```python
from build123d import *

# Parameters (mm, degrees)
SKETCH1_R           = 124
BOSS_EXTRUDE1_DEPTH = 6.35
SKETCH6_R           = 2.5527
CUT_EXTRUDE1_DEPTH  = 176.477413076
SKETCH8_R           = 11
CUT_EXTRUDE3_DEPTH  = 176.477413076
SKETCH9_R           = 2.45
CUT_EXTRUDE4_DEPTH  = 176.477413076
SKETCH12_R          = 1.45
CUT_EXTRUDE5_DEPTH  = 176.477413076
SKETCH13_R          = 54
CUT_EXTRUDE6_DEPTH  = 176.477413076


with BuildPart() as part:
    # Sketch1 → Boss-Extrude1 (new body)
    with BuildSketch(Plane(origin=(0, 0, 0), x_dir=(1, 0, 0), z_dir=(0, 1, 0))):
        with Locations(Location((0, 0, 0), (0, 0, 270))):
            Circle(SKETCH1_R)
    extrude(amount=BOSS_EXTRUDE1_DEPTH)

    # Sketch6 → Cut-Extrude1 (cut, through all)
    with BuildSketch(Plane.XZ):
        with Locations(Location((-109.204648421, 41.27165811, 0), (0, 0, 270))):
            Circle(SKETCH6_R)
        with Locations(Location((-106.602870566, -47.590261473, 0), (0, 0, 270))):
            Circle(SKETCH6_R)
        with Locations(Location((109.204648421, -41.27165811, 0), (0, 0, 270))):
            Circle(SKETCH6_R)
        with Locations(Location((106.602870566, 47.590261473, 0), (0, 0, 270))):
            Circle(SKETCH6_R)
        with Locations(Location((41.27165811, 109.204648421, 0), (0, 0, 270))):
            Circle(SKETCH6_R)
        with Locations(Location((-47.590261473, 106.602870566, 0), (0, 0, 270))):
            Circle(SKETCH6_R)
        with Locations(Location((-41.27165811, -109.204648421, 0), (0, 0, 270))):
            Circle(SKETCH6_R)
        with Locations(Location((47.590261473, -106.602870566, 0), (0, 0, 270))):
            Circle(SKETCH6_R)
    extrude(amount=-CUT_EXTRUDE1_DEPTH, mode=Mode.SUBTRACT)

    # Sketch8 → Cut-Extrude3 (cut, through all)
    with BuildSketch(Plane(origin=(0, 6.35, 0), x_dir=(1, 0, 0), z_dir=(0, 1, 0))):
        with Locations(Location((0, 0, 0), (0, 0, 270))):
            Circle(SKETCH8_R)
    extrude(amount=-CUT_EXTRUDE3_DEPTH, mode=Mode.SUBTRACT)

    # Sketch9 → Cut-Extrude4 (cut, through all)
    with BuildSketch(Plane(origin=(0, 6.35, 0), x_dir=(1, 0, 0), z_dir=(0, 1, 0))):
        with Locations(Location((-15.112143296, -8.725, 0), (0, 0, 270))):
            Circle(SKETCH9_R)
        with Locations(Location((0, 17.45, 0), (0, 0, 270))):
            Circle(SKETCH9_R)
        with Locations(Location((15.112143296, -8.725, 0), (0, 0, 270))):
            Circle(SKETCH9_R)
    extrude(amount=-CUT_EXTRUDE4_DEPTH, mode=Mode.SUBTRACT)

    # Sketch12 → Cut-Extrude5 (cut, through all)
    with BuildSketch(Plane(origin=(0, 6.35, 0), x_dir=(1, 0, 0), z_dir=(0, 1, 0))):
        with Locations(Location((0, 30, 0), (0, 0, 270))):
            Circle(SKETCH12_R)
        with Locations(Location((0, 60, 0), (0, 0, 270))):
            Circle(SKETCH12_R)
        with Locations(Location((0, 90, 0), (0, 0, 270))):
            Circle(SKETCH12_R)
        with Locations(Location((11.480502971, 27.716385975, 0), (0, 0, 270))):
            Circle(SKETCH12_R)
        with Locations(Location((21.213203436, 21.213203436, 0), (0, 0, 270))):
            Circle(SKETCH12_R)
        with Locations(Location((27.716385975, 11.480502971, 0), (0, 0, 270))):
            Circle(SKETCH12_R)
        with Locations(Location((30, 0, 0), (0, 0, 270))):
            Circle(SKETCH12_R)
        with Locations(Location((27.716385975, -11.480502971, 0), (0, 0, 270))):
            Circle(SKETCH12_R)
        with Locations(Location((21.213203436, -21.213203436, 0), (0, 0, 270))):
            Circle(SKETCH12_R)
        with Locations(Location((11.480502971, -27.716385975, 0), (0, 0, 270))):
            Circle(SKETCH12_R)
        with Locations(Location((0, -30, 0), (0, 0, 270))):
            Circle(SKETCH12_R)
        with Locations(Location((-11.480502971, -27.716385975, 0), (0, 0, 270))):
            Circle(SKETCH12_R)
        with Locations(Location((-21.213203436, -21.213203436, 0), (0, 0, 270))):
            Circle(SKETCH12_R)
        with Locations(Location((-27.716385975, -11.480502971, 0), (0, 0, 270))):
            Circle(SKETCH12_R)
        with Locations(Location((-30, 0, 0), (0, 0, 270))):
            Circle(SKETCH12_R)
        with Locations(Location((-27.716385975, 11.480502971, 0), (0, 0, 270))):
            Circle(SKETCH12_R)
        with Locations(Location((-21.213203436, 21.213203436, 0), (0, 0, 270))):
            Circle(SKETCH12_R)
        with Locations(Location((-11.480502971, 27.716385975, 0), (0, 0, 270))):
            Circle(SKETCH12_R)
        with Locations(Location((11.705419321, 58.847116824, 0), (0, 0, 270))):
            Circle(SKETCH12_R)
        with Locations(Location((22.961005942, 55.432771951, 0), (0, 0, 270))):
            Circle(SKETCH12_R)
        with Locations(Location((33.334213981, 49.888176738, 0), (0, 0, 270))):
            Circle(SKETCH12_R)
        with Locations(Location((42.426406871, 42.426406871, 0), (0, 0, 270))):
            Circle(SKETCH12_R)
        with Locations(Location((49.888176738, 33.334213981, 0), (0, 0, 270))):
            Circle(SKETCH12_R)
        with Locations(Location((55.432771951, 22.961005942, 0), (0, 0, 270))):
            Circle(SKETCH12_R)
        with Locations(Location((58.847116824, 11.705419321, 0), (0, 0, 270))):
            Circle(SKETCH12_R)
        with Locations(Location((60, 0, 0), (0, 0, 270))):
            Circle(SKETCH12_R)
        with Locations(Location((58.847116824, -11.705419321, 0), (0, 0, 270))):
            Circle(SKETCH12_R)
        with Locations(Location((55.432771951, -22.961005942, 0), (0, 0, 270))):
            Circle(SKETCH12_R)
        with Locations(Location((49.888176738, -33.334213981, 0), (0, 0, 270))):
            Circle(SKETCH12_R)
        with Locations(Location((42.426406871, -42.426406871, 0), (0, 0, 270))):
            Circle(SKETCH12_R)
        with Locations(Location((33.334213981, -49.888176738, 0), (0, 0, 270))):
            Circle(SKETCH12_R)
        with Locations(Location((22.961005942, -55.432771951, 0), (0, 0, 270))):
            Circle(SKETCH12_R)
        with Locations(Location((11.705419321, -58.847116824, 0), (0, 0, 270))):
            Circle(SKETCH12_R)
        with Locations(Location((0, -60, 0), (0, 0, 270))):
            Circle(SKETCH12_R)
        with Locations(Location((-11.705419321, -58.847116824, 0), (0, 0, 270))):
            Circle(SKETCH12_R)
        with Locations(Location((-22.961005942, -55.432771951, 0), (0, 0, 270))):
            Circle(SKETCH12_R)
        with Locations(Location((-33.334213981, -49.888176738, 0), (0, 0, 270))):
            Circle(SKETCH12_R)
        with Locations(Location((-42.426406871, -42.426406871, 0), (0, 0, 270))):
            Circle(SKETCH12_R)
        with Locations(Location((-49.888176738, -33.334213981, 0), (0, 0, 270))):
            Circle(SKETCH12_R)
        with Locations(Location((-55.432771951, -22.961005942, 0), (0, 0, 270))):
            Circle(SKETCH12_R)
        with Locations(Location((-58.847116824, -11.705419321, 0), (0, 0, 270))):
            Circle(SKETCH12_R)
        with Locations(Location((-60, 0, 0), (0, 0, 270))):
            Circle(SKETCH12_R)
        with Locations(Location((-58.847116824, 11.705419321, 0), (0, 0, 270))):
            Circle(SKETCH12_R)
        with Locations(Location((-55.432771951, 22.961005942, 0), (0, 0, 270))):
            Circle(SKETCH12_R)
        with Locations(Location((-49.888176738, 33.334213981, 0), (0, 0, 270))):
            Circle(SKETCH12_R)
        with Locations(Location((-42.426406871, 42.426406871, 0), (0, 0, 270))):
            Circle(SKETCH12_R)
        with Locations(Location((-33.334213981, 49.888176738, 0), (0, 0, 270))):
            Circle(SKETCH12_R)
        with Locations(Location((-22.961005942, 55.432771951, 0), (0, 0, 270))):
            Circle(SKETCH12_R)
        with Locations(Location((-11.705419321, 58.847116824, 0), (0, 0, 270))):
            Circle(SKETCH12_R)
        with Locations(Location((14.079101854, 88.891950654, 0), (0, 0, 270))):
            Circle(SKETCH12_R)
        with Locations(Location((27.811529494, 85.595086467, 0), (0, 0, 270))):
            Circle(SKETCH12_R)
        with Locations(Location((40.859144977, 80.190587177, 0), (0, 0, 270))):
            Circle(SKETCH12_R)
        with Locations(Location((52.900672706, 72.811529494, 0), (0, 0, 270))):
            Circle(SKETCH12_R)
        with Locations(Location((63.639610307, 63.639610307, 0), (0, 0, 270))):
            Circle(SKETCH12_R)
        with Locations(Location((72.811529494, 52.900672706, 0), (0, 0, 270))):
            Circle(SKETCH12_R)
        with Locations(Location((80.190587177, 40.859144977, 0), (0, 0, 270))):
            Circle(SKETCH12_R)
        with Locations(Location((85.595086467, 27.811529494, 0), (0, 0, 270))):
            Circle(SKETCH12_R)
        with Locations(Location((88.891950654, 14.079101854, 0), (0, 0, 270))):
            Circle(SKETCH12_R)
        with Locations(Location((90, 0, 0), (0, 0, 270))):
            Circle(SKETCH12_R)
        with Locations(Location((88.891950654, -14.079101854, 0), (0, 0, 270))):
            Circle(SKETCH12_R)
        with Locations(Location((85.595086467, -27.811529494, 0), (0, 0, 270))):
            Circle(SKETCH12_R)
        with Locations(Location((80.190587177, -40.859144977, 0), (0, 0, 270))):
            Circle(SKETCH12_R)
        with Locations(Location((72.811529494, -52.900672706, 0), (0, 0, 270))):
            Circle(SKETCH12_R)
        with Locations(Location((63.639610307, -63.639610307, 0), (0, 0, 270))):
            Circle(SKETCH12_R)
        with Locations(Location((52.900672706, -72.811529494, 0), (0, 0, 270))):
            Circle(SKETCH12_R)
        with Locations(Location((40.859144977, -80.190587177, 0), (0, 0, 270))):
            Circle(SKETCH12_R)
        with Locations(Location((27.811529494, -85.595086467, 0), (0, 0, 270))):
            Circle(SKETCH12_R)
        with Locations(Location((14.079101854, -88.891950654, 0), (0, 0, 270))):
            Circle(SKETCH12_R)
        with Locations(Location((0, -90, 0), (0, 0, 270))):
            Circle(SKETCH12_R)
        with Locations(Location((-14.079101854, -88.891950654, 0), (0, 0, 270))):
            Circle(SKETCH12_R)
        with Locations(Location((-27.811529494, -85.595086467, 0), (0, 0, 270))):
            Circle(SKETCH12_R)
        with Locations(Location((-40.859144977, -80.190587177, 0), (0, 0, 270))):
            Circle(SKETCH12_R)
        with Locations(Location((-52.900672706, -72.811529494, 0), (0, 0, 270))):
            Circle(SKETCH12_R)
        with Locations(Location((-63.639610307, -63.639610307, 0), (0, 0, 270))):
            Circle(SKETCH12_R)
        with Locations(Location((-72.811529494, -52.900672706, 0), (0, 0, 270))):
            Circle(SKETCH12_R)
        with Locations(Location((-80.190587177, -40.859144977, 0), (0, 0, 270))):
            Circle(SKETCH12_R)
        with Locations(Location((-85.595086467, -27.811529494, 0), (0, 0, 270))):
            Circle(SKETCH12_R)
        with Locations(Location((-88.891950654, -14.079101854, 0), (0, 0, 270))):
            Circle(SKETCH12_R)
        with Locations(Location((-90, 0, 0), (0, 0, 270))):
            Circle(SKETCH12_R)
        with Locations(Location((-88.891950654, 14.079101854, 0), (0, 0, 270))):
            Circle(SKETCH12_R)
        with Locations(Location((-85.595086467, 27.811529494, 0), (0, 0, 270))):
            Circle(SKETCH12_R)
        with Locations(Location((-80.190587177, 40.859144977, 0), (0, 0, 270))):
            Circle(SKETCH12_R)
        with Locations(Location((-72.811529494, 52.900672706, 0), (0, 0, 270))):
            Circle(SKETCH12_R)
        with Locations(Location((-63.639610307, 63.639610307, 0), (0, 0, 270))):
            Circle(SKETCH12_R)
        with Locations(Location((-52.900672706, 72.811529494, 0), (0, 0, 270))):
            Circle(SKETCH12_R)
        with Locations(Location((-40.859144977, 80.190587177, 0), (0, 0, 270))):
            Circle(SKETCH12_R)
        with Locations(Location((-27.811529494, 85.595086467, 0), (0, 0, 270))):
            Circle(SKETCH12_R)
        with Locations(Location((-14.079101854, 88.891950654, 0), (0, 0, 270))):
            Circle(SKETCH12_R)
    extrude(amount=-CUT_EXTRUDE5_DEPTH, mode=Mode.SUBTRACT)

    # Sketch13 → Cut-Extrude6 (cut, through all)
    with BuildSketch(Plane(origin=(0, 6.35, 0), x_dir=(1, 0, 0), z_dir=(0, 1, 0))):
        with Locations(Location((0, 0, 0), (0, 0, 270))):
            Circle(SKETCH13_R)
    extrude(amount=-CUT_EXTRUDE6_DEPTH, mode=Mode.SUBTRACT)


solid = part.part
```
Geometry check sheet. Reference: the model listing, model coordinates, mm. Coordinates: 2 decimals unless noted, no trailing zeros. Loops run counter-clockwise (first coordinate to the right, second up) from the corner with the lowest first, then second, coordinate; pieces in that order, holes last. Notation, with made-up numbers: (26, 53.25) - (47, 53.25) arc R10 cw to (47, 62.25) - close; hole circle Ø6 at (-31, 83.25). An arc over 180 degrees is marked (long way). One line per item, written item: value. Start each with the question number.
(1) Cross-section at A-A on y = 3. Count the separate pieces of the cut face and the enclosed holes in it, plus the area to 3 significant figures.
(2) Cross-section at B-B on x = -101. Enter the section's corners in (y, z).
(3) Depth check by flat-ended pin: P1, Ø12, axis at x = 43, z = 17, coming from the +Y side; P2, Ø1.5, axis at x = 51, y = 5, coming from the +Z side; P3, Ø2, axis at x = -81, y = 3, coming from the -Z side; P4, Ø2, axis at y = 2.5, z = -17.5, coming from the -X side. Enter the tip coordinate at first touch or a pass-through.
(4) Material ranges on line 1 (Z direction, x = 28.5, y = 5); line 2 (Z direction, x = 55.5, y = 2.75); line 3 (X direction, y = 6, z = -88.5), recorded low to high. Write a range as [from, to].
(5) Mould release check, pull along X, two halves, no side actions. Record for faces 1 (the cylindrical face through (122.945, 3.131, -16.142)), 2 (the cylindrical face through (-52.716, 3.219, -11.706)), 3 (the flat face through (-26, 6.35, 53)): released by +X, released by -X, zero draft, split by the parting line, or undercut.
Results below:
1. separate pieces: 1
1. enclosed holes: 81
1. area: 38,500 mm2
2. outline: (0, -71.94) - (6.35, -71.94) - (6.35, 71.94) - (0, 71.94) - close
3. P1: passes through
3. P2: stops at z = 113.36
3. P3: stops at z = -94.74
3. P4: stops at x = -122.9
4. line 1: z = [-120.68, -86.87], [-84.32, -45.87], [45.87, 84.32], [86.87, 120.68]
4. line 2: z = [-110.89, -24.41], [-21.51, 21.51], [24.41, 110.89]
4. line 3: x = [-86.85, -15.48], [-12.68, 12.68], [15.48, 86.85]
5. face 1: split by the parting line
5. face 2: undercut
5. face 3: zero draft
